from build123d import *

# Parameters (mm, degrees)
BOSS_EXTRUDE1_DEPTH           = 15
BOSS_EXTRUDE2_DEPTH           = 5
SKETCH3_R                     = 11
CUT_EXTRUDE1_DEPTH            = 7.1
CUT_EXTRUDE2_REACH            = 75.61
SKETCH4_R                     = 7
FILLET1_R                     = 5
FILLET2_R                     = 5
FILLET3_R                     = 1
FILLET6_START                 = -30
FILLET6_DEPTH                 = 6.9999999
FILLET6_2_ANGLE               = 90
FILLET6_3_ANGLE               = 90
CSK_FOR_M4_SFHCS1_D           = 4.5
CSK_FOR_M4_SFHCS1_CSINK_D     = 8.96
CSK_FOR_M4_SFHCS1_CSINK_ANGLE = 90


with BuildPart() as part:
    # Sketch2 → Boss-Extrude1 (new, symmetric)
    with BuildSketch(Plane(origin=(0, 0, 0), x_dir=(1, 0, 0), z_dir=(0, 1, 0))):
        Polygon((-35, 22), (0, 22), (0, -22), (-35, -22), (-35, -30), (5, -30), (5, 30), (-35, 30), align=None)
    extrude(amount=BOSS_EXTRUDE1_DEPTH, both=True)

    # Sketch5 → Boss-Extrude2 (add)
    with BuildSketch(Plane(origin=(5, 0, 0), x_dir=(0, 0, -1), z_dir=(1, 0, 0))):
        Polygon((-10, 37.35), (30, 37.35), (30, -30), (-10, -30), (-10, -15), (-30, -15), (-30, 15), (-10, 15), align=None)
    extrude(amount=-BOSS_EXTRUDE2_DEPTH)

    # Sketch3 → Cut-Extrude1 (cut)
    with BuildSketch(Plane(origin=(0, 0, -30), x_dir=(-1, 0, 0), z_dir=(0, 0, -1))):
        with Locations((21, 0)):
            Circle(SKETCH3_R)
    cut_extrude1 = extrude(amount=-CUT_EXTRUDE1_DEPTH, mode=Mode.SUBTRACT)

    # Sketch4 → Cut-Extrude2 (cut, up to next)
    with BuildSketch(Plane(origin=(0, 0, -22.9), x_dir=(-1, 0, 0), z_dir=(0, 0, -1)), mode=Mode.PRIVATE) as cut_extrude2_sk1:
        with Locations((21, 0)):
            Circle(SKETCH4_R)
    cut_extrude2_tool1 = extrude(cut_extrude2_sk1.sketch, amount=-CUT_EXTRUDE2_REACH, mode=Mode.PRIVATE) & part.part
    cut_extrude2 = cut_extrude2_tool1.solids().sort_by_distance((-21, 0, -22.9))[0]
    add(cut_extrude2, mode=Mode.SUBTRACT)

    # Mirror1: Cut-Extrude1, Cut-Extrude2 across plane
    add(cut_extrude1.mirror(Plane.XY), mode=Mode.SUBTRACT)
    add(cut_extrude2.mirror(Plane.XY), mode=Mode.SUBTRACT)

    # Fillet1
    fillet1_edges = [part.edges().sort_by_distance(p)[0] for p in [
        (0, 0, 22),
        (0, 0, -22),
    ]]
    fillet(fillet1_edges, radius=FILLET1_R)

    # Fillet2
    fillet2_edges = [part.edges().sort_by_distance(p)[0] for p in [
        (-35, -15, -26),
        (-35, 15, 26),
        (2.5, -15, 10),
        (2.5, 15, 10),
        (-35, 15, -26),
        (-35, -15, 26),
    ]]
    fillet(fillet2_edges, radius=FILLET2_R)

    # Fillet3
    # the kernel refuses this fillet: 1 mm, written as the material it takes off along each edge
    with BuildSketch(Plane(origin=(-5, 15, 17), x_dir=(1, 0, 0), z_dir=(0, 0, -1))) as fillet3_piece_1:
        with BuildLine():
            CenterArc((5 + FILLET3_R, FILLET3_R), FILLET3_R, 180, 90)
            Line((5 + FILLET3_R, 0), (5, 0))
            Line((5, 0), (5, FILLET3_R))
        make_face()
    revolve(axis=Axis((-5, 15, 17), (0, -1, 0)), revolution_arc=90, mode=Mode.SUBTRACT)
    with BuildSketch(Plane(origin=(-5, 15, -17), x_dir=(0, 0, -1), z_dir=(-1, 0, 0))) as fillet3_piece_2_section:
        with BuildLine():
            CenterArc((5 + FILLET3_R, FILLET3_R), FILLET3_R, 180, 90)
            Line((5 + FILLET3_R, 0), (5, 0))
            Line((5, 0), (5, FILLET3_R))
        make_face()
    fillet3_piece_2 = revolve(axis=Axis((-5, 15, -17), (0, -1, 0)), revolution_arc=138.720976341, mode=Mode.PRIVATE)
    fillet3_piece_2 = split(fillet3_piece_2, bisect_by=Plane(origin=(0, 15, -17), z_dir=(-1, 0, 0)), keep=Keep.TOP, mode=Mode.PRIVATE)
    add(fillet3_piece_2, mode=Mode.SUBTRACT)
    with BuildSketch(Plane(origin=(-30, 15, -22), x_dir=(0, -1, 0), z_dir=(1, 0, 0)), Plane(origin=(-5, -15, 22), x_dir=(0, 0, 1), z_dir=(-1, 0, 0))) as fillet3_piece_3:
        with BuildLine():
            CenterArc((FILLET3_R, FILLET3_R), FILLET3_R, 180, 90)
            Line((0, FILLET3_R), (0, 0))
            Line((0, 0), (FILLET3_R, 0))
        make_face()
    extrude(amount=25, mode=Mode.SUBTRACT)
    with BuildSketch(Plane(origin=(-30, 10, -22), x_dir=(0, 1, 0), z_dir=(1, 0, 0))) as fillet3_piece_4:
        with BuildLine():
            CenterArc((5 - FILLET3_R, -FILLET3_R), FILLET3_R, 0, 90)
            Line((5, -FILLET3_R), (5, 0))
            Line((5, 0), (5 - FILLET3_R, 0))
        make_face()
    revolve(axis=Axis((-30, 10, -22), (0, 0, 1)), revolution_arc=90, mode=Mode.SUBTRACT)
    with BuildSketch(Plane(origin=(-35, 10, -22), x_dir=(1, 0, 0), z_dir=(0, -1, 0)), Plane(origin=(-35, -10, 22), x_dir=(1, 0, 0), z_dir=(0, 1, 0))) as fillet3_piece_5:
        with BuildLine():
            CenterArc((FILLET3_R, -FILLET3_R), FILLET3_R, 90, 90)
            Line((0, -FILLET3_R), (0, 0))
            Line((0, 0), (FILLET3_R, 0))
        make_face()
    extrude(amount=20, mode=Mode.SUBTRACT)
    with BuildSketch(Plane(origin=(-30, -10, -22), x_dir=(-1, 0, 0), z_dir=(0, 1, 0))) as fillet3_piece_6:
        with BuildLine():
            CenterArc((5 - FILLET3_R, -FILLET3_R), FILLET3_R, 0, 90)
            Line((5, -FILLET3_R), (5, 0))
            Line((5, 0), (5 - FILLET3_R, 0))
        make_face()
    revolve(axis=Axis((-30, -10, -22), (0, 0, 1)), revolution_arc=90, mode=Mode.SUBTRACT)
    with BuildSketch(Plane(origin=(-30, -15, -22), x_dir=(0, 1, 0), z_dir=(1, 0, 0)), Plane(origin=(-5, 15, 22), x_dir=(0, 0, 1), z_dir=(-1, 0, 0))) as fillet3_piece_7:
        with BuildLine():
            CenterArc((FILLET3_R, -FILLET3_R), FILLET3_R, 90, 90)
            Line((0, -FILLET3_R), (0, 0))
            Line((0, 0), (FILLET3_R, 0))
        make_face()
    extrude(amount=25, mode=Mode.SUBTRACT)
    with BuildSketch(Plane(origin=(-5, -15, -17), x_dir=(0, 0, -1), z_dir=(-1, 0, 0))) as fillet3_piece_8_section:
        with BuildLine():
            CenterArc((5 + FILLET3_R, -FILLET3_R), FILLET3_R, 90, 90)
            Line((5, -FILLET3_R), (5, 0))
            Line((5, 0), (5 + FILLET3_R, 0))
        make_face()
    fillet3_piece_8 = revolve(axis=Axis((-5, -15, -17), (0, -1, 0)), revolution_arc=138.720976341, mode=Mode.PRIVATE)
    fillet3_piece_8 = split(fillet3_piece_8, bisect_by=Plane(origin=(0, -15, -17), z_dir=(-1, 0, 0)), keep=Keep.TOP, mode=Mode.PRIVATE)
    add(fillet3_piece_8, mode=Mode.SUBTRACT)
    with BuildSketch(Plane(origin=(-5, -15, 17), x_dir=(1, 0, 0), z_dir=(0, 0, -1))) as fillet3_piece_9:
        with BuildLine():
            CenterArc((5 + FILLET3_R, -FILLET3_R), FILLET3_R, 90, 90)
            Line((5, -FILLET3_R), (5, 0))
            Line((5, 0), (5 + FILLET3_R, 0))
        make_face()
    revolve(axis=Axis((-5, -15, 17), (0, -1, 0)), revolution_arc=90, mode=Mode.SUBTRACT)
    with BuildSketch(Plane(origin=(-30, -10, 22), x_dir=(0, -1, 0), z_dir=(1, 0, 0))) as fillet3_piece_10:
        with BuildLine():
            CenterArc((5 - FILLET3_R, -FILLET3_R), FILLET3_R, 0, 90)
            Line((5, -FILLET3_R), (5, 0))
            Line((5, 0), (5 - FILLET3_R, 0))
        make_face()
    revolve(axis=Axis((-30, -10, 22), (0, 0, -1)), revolution_arc=90, mode=Mode.SUBTRACT)
    with BuildSketch(Plane(origin=(-30, 10, 22), x_dir=(0, 1, 0), z_dir=(1, 0, 0))) as fillet3_piece_11:
        with BuildLine():
            CenterArc((5 - FILLET3_R, FILLET3_R), FILLET3_R, 270, 90)
            Line((5, FILLET3_R), (5, 0))
            Line((5, 0), (5 - FILLET3_R, 0))
        make_face()
    revolve(axis=Axis((-30, 10, 22), (0, 0, 1)), revolution_arc=90, mode=Mode.SUBTRACT)
    with BuildSketch(Plane(origin=(0, 15, 15), x_dir=(0, -1, 0), z_dir=(0, 0, 1))) as fillet3_piece_12:
        with BuildLine():
            CenterArc((FILLET3_R, FILLET3_R), FILLET3_R, 180, 90)
            Line((0, FILLET3_R), (0, 0))
            Line((0, 0), (FILLET3_R, 0))
        make_face()
    extrude(amount=2, mode=Mode.SUBTRACT)
    with BuildSketch(Plane(origin=(0, -15, 15), x_dir=(0, 1, 0), z_dir=(0, 0, 1))) as fillet3_piece_13:
        with BuildLine():
            CenterArc((FILLET3_R, -FILLET3_R), FILLET3_R, 90, 90)
            Line((0, -FILLET3_R), (0, 0))
            Line((0, 0), (FILLET3_R, 0))
        make_face()
    extrude(amount=2, mode=Mode.SUBTRACT)
    with BuildSketch(Plane(origin=(0, 20, 10), x_dir=(0, 0, -1), z_dir=(0, 1, 0))) as fillet3_piece_14:
        with BuildLine():
            CenterArc((FILLET3_R, -FILLET3_R), FILLET3_R, 90, 90)
            Line((0, -FILLET3_R), (0, 0))
            Line((0, 0), (FILLET3_R, 0))
        make_face()
    extrude(amount=19.85, mode=Mode.SUBTRACT)
    with BuildSketch(Plane(origin=(0, 20, 15), x_dir=(0, -1, 0), z_dir=(0, 0, 1))) as fillet3_piece_15:
        with BuildLine():
            CenterArc((5 + FILLET3_R, FILLET3_R), FILLET3_R, 180, 90)
            Line((5, FILLET3_R), (5, 0))
            Line((5, 0), (5 + FILLET3_R, 0))
        make_face()
    revolve(axis=Axis((0, 20, 15), (1, 0, 0)), revolution_arc=90, mode=Mode.SUBTRACT)
    with BuildSketch(Plane(origin=(0, -32.5, 10), x_dir=(0, 0, -1), z_dir=(0, 1, 0))) as fillet3_piece_16:
        with BuildLine():
            CenterArc((FILLET3_R, -FILLET3_R), FILLET3_R, 90, 90)
            Line((0, -FILLET3_R), (0, 0))
            Line((0, 0), (FILLET3_R, 0))
        make_face()
    extrude(amount=12.5, mode=Mode.SUBTRACT)
    with BuildSketch(Plane(origin=(0, -20, 15), x_dir=(0, 0, -1), z_dir=(0, -1, 0))) as fillet3_piece_17:
        with BuildLine():
            CenterArc((5 + FILLET3_R, FILLET3_R), FILLET3_R, 180, 90)
            Line((5, FILLET3_R), (5, 0))
            Line((5, 0), (5 + FILLET3_R, 0))
        make_face()
    revolve(axis=Axis((0, -20, 15), (1, 0, 0)), revolution_arc=90, mode=Mode.SUBTRACT)

    # Fillet6: read off the stored shape, not the designer's step
    # Fillet6 outline → Fillet6 (add)
    with BuildSketch(Plane.XY.offset(FILLET6_START)):
        with BuildLine():
            Line((-5, 15), (0, 15))
            Line((0, 15), (0, 20))
            ThreePointArc((0, 20), (-1.464466094, 16.464466094), (-5, 15))
        make_face()
        with BuildLine():
            ThreePointArc((-5, -15), (-1.464466094, -16.464466094), (0, -20))
            Line((0, -20), (0, -15))
            Line((0, -15), (-5, -15))
        make_face()
    extrude(amount=FILLET6_DEPTH)

    # Fillet6 2 outline → Fillet6 2 (revolve)
    with BuildSketch(Plane(origin=(0, -14, -23), x_dir=(0, 0, 1), z_dir=(0, 1, 0))):
        with BuildLine():
            ThreePointArc((1, -5), (2.464466094, -1.464466094), (6, 0))
            Line((6, 0), (1, 0))
            Line((1, 0), (1, -5))
        make_face()
    revolve(axis=Axis((0, -14, -23), (1, 0, 0)), revolution_arc=FILLET6_2_ANGLE)

    # Fillet6 3 outline → Fillet6 3 (revolve)
    with BuildSketch(Plane(origin=(0, 14, -23), x_dir=(0, 1, 0), z_dir=(0, 0, -1))):
        with BuildLine():
            ThreePointArc((1, -5), (2.464466094, -1.464466094), (6, 0))
            Line((6, 0), (1, 0))
            Line((1, 0), (1, -5))
        make_face()
    revolve(axis=Axis((0, 14, -23), (1, 0, 0)), revolution_arc=FILLET6_3_ANGLE)

    # CSK for M4 SFHCS1 (through all)
    with Locations(Plane.ZY):
        with Locations((0, 32.35), (-20, -25), (0, -25), (-20, 32.35)):
            CounterSinkHole(CSK_FOR_M4_SFHCS1_D / 2, CSK_FOR_M4_SFHCS1_CSINK_D / 2, counter_sink_angle=CSK_FOR_M4_SFHCS1_CSINK_ANGLE)


solid = part.part
Can you work these out from the model? Positions are in its coordinate system, mm. A direction names the side the tool comes from. Coordinates: 2 decimals unless noted, no trailing zeros. Write each loop counter-clockwise with the first axis right and the second up, starting at its lowest first coordinate (ties: lowest second). Pieces come first, ordered by that corner, then holes. Notation, with made-up numbers: (33, 78.25) -> (44, 78.25) arc R25 ccw to (44, 107.25) -> close; hole circle Ø3 at (-35, 62.5). An arc over 180 degrees is marked (long way). Write each question's results on one line, items separated by ' | '. Start each with the question number.
Item 1: If we section it at A-A, the plane y = 32.35: Write out the boundary of the cut face in (x, z).
Item 2: If we section it at D-D, the plane x = -13: Write out the boundary of the cut face in (y, z), and give its area (3 significant figures).
Item 3: If we section it at B-B, the plane x = -21: Write out the boundary of the cut face in (y, z).
Item 4: On a 3-axis mill with a long thin cutter (end or side, diameter ignored), from which of +Z, -Z, +X, -X, +Y, -Y can I reach the whole of each face in a straight line? I mean faces 1 (the flat face through (-18, -15, -27)), 2 (the flat face through (-18, 15, -27)), 3 (the flat face through (3, 29, 10)), 4 (the cylindrical face through (-31.161, -4.213, -26.5)), 5 (the cylindrical face through (-1, 0, 20)). Say none if no direction works.
Item 5: If we section it at C-C, the plane z = 0: Write out the boundary of the cut face in (x, y).
Item 6: Please list where these lines run through material, in increasing order: probe 1 along Z at (x, y) = (2.9, -25); probe 2 along Z at (x, y) = (-11, 5); probe 3 along Y at (x, z) = (-21, 27.25).
Item 7: Thinking about a two-plate mould opening in Z: for faces 6 (the flat face through (-28.2, 0.2, -22.9)), 7 (the conical face through (2.122, -27.092, -1.088)), 8 (the flat face through (-35, 0, 26)), which applies, released by +Z, released by -Z, zero draft, split by the parting line, or undercut?
Item 8: I'm going to push flat-ended pins straight in: P1, Ø1, axis at x = -28, y = 7.5, coming from the +Z side; P2, Ø2, axis at x = 3, y = 31, coming from the +Z side; P3, Ø3.5, axis at x = -19, z = -27.5, coming from the +Y side. Where does each tip first touch, or does it pass through?
Answer block:
1) outline: (0, -30) -> (5, -30) -> (5, -22.25) -> (2.23, -22.25) -> (0, -24.48) -> close; (0, -15.52) -> (2.23, -17.75) -> (5, -17.75) -> (5, -2.25) -> (2.23, -2.25) -> (0, -4.48) -> close; (0, 4.48) -> (2.23, 2.25) -> (5, 2.25) -> (5, 10) -> (1, 10) arc R1 ccw to (0, 9) -> close
2) outline: (-15, -30) -> (-7.55, -30) -> (-7.55, -22.9) -> (7.55, -22.9) -> (7.55, -30) -> (15, -30) -> (15, -23) arc R1 ccw to (14, -22) -> (-14, -22) arc R1 ccw to (-15, -23) -> close; (-15, 23) arc R1 ccw to (-14, 22) -> (14, 22) arc R1 ccw to (15, 23) -> (15, 30) -> (7.55, 30) -> (7.55, 22.9) -> (-7.55, 22.9) -> (-7.55, 30) -> (-15, 30) -> close | area: 265 mm²
3) outline: (-15, -30) -> (-11, -30) -> (-11, -22.9) -> (-7, -22.9) -> (-7, -22) -> (-14, -22) arc R1 ccw to (-15, -23) -> close; (-15, 23) arc R1 ccw to (-14, 22) -> (-7, 22) -> (-7, 22.9) -> (-11, 22.9) -> (-11, 30) -> (-15, 30) -> close; (7, -22.9) -> (11, -22.9) -> (11, -30) -> (15, -30) -> (15, -23) arc R1 ccw to (14, -22) -> (7, -22) -> close; (7, 22) -> (14, 22) arc R1 ccw to (15, 23) -> (15, 30) -> (11, 30) -> (11, 22.9) -> (7, 22.9) -> close
4) face 1: +Z, -Z, -X, -Y | face 2: +Z, -Z, -X, +Y | face 3: +Z, +X, -X, +Y | face 4: -Z | face 5: -X, +Y, -Y
5) outline: (0, -30) -> (5, -30) -> (5, -27.25) -> (2.23, -27.25) -> (0, -29.48) -> close; (0, -20.52) -> (2.23, -22.75) -> (5, -22.75) -> (5, 30.1) -> (2.23, 30.1) -> (0, 27.87) -> close; (0, 36.83) -> (2.23, 34.6) -> (5, 34.6) -> (5, 37.35) -> (0, 37.35) -> close
6) probe 1: -30 to -22.25, -17.75 to -2.25, 2.25 to 10 | probe 2: -30 to -22, 22 to 30 | probe 3: -15 to -11, 11 to 15
7) face 6: released by -Z | face 7: undercut | face 8: zero draft
8) P1: z = 22.9 | P2: z = 10 | P3: y = 15
